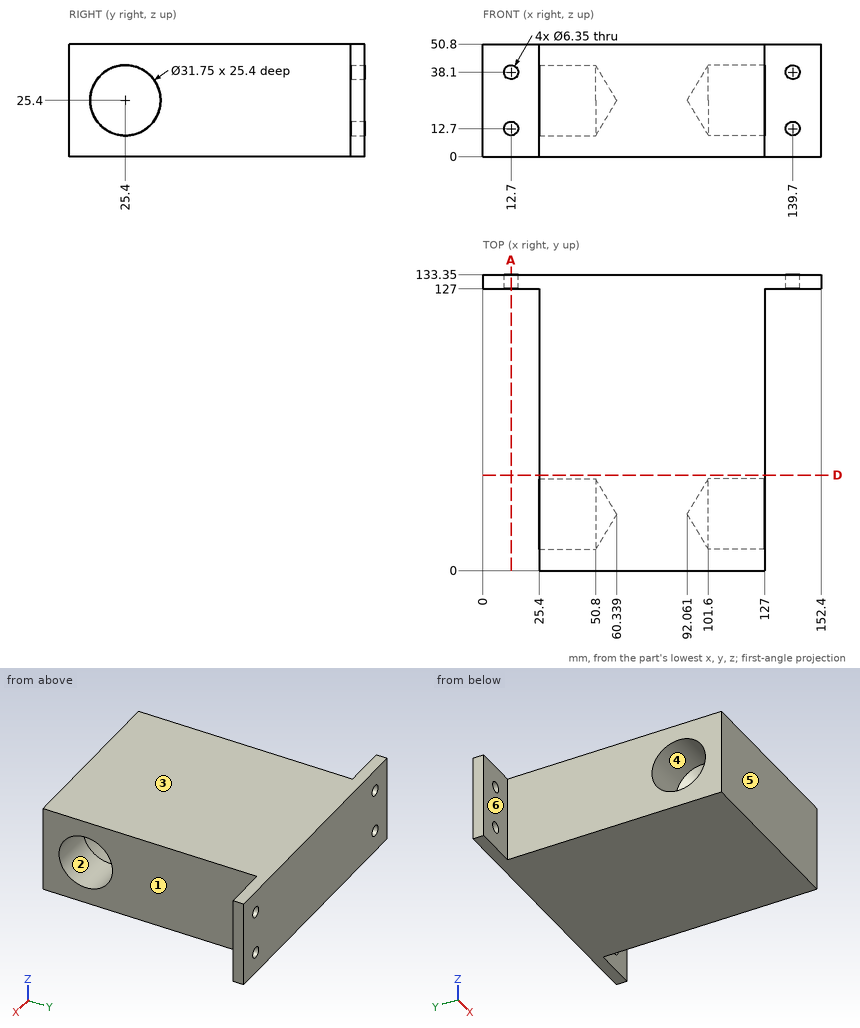
Design review of the part shown in the three views and the two pictorial views. Dimensions are in mm from the part's minimum x, y and z. A direction names the side the tool comes from. Round coordinates to 2 decimals unless told otherwise and drop trailing zeros. Order: outer loops, then holes, each group sorted by start corner. A loop starts at its lowest first (then second) coordinate and runs counter-clockwise, first axis right, second up.
(1) Take a section at A-A, the plane x = 12.7. Count the separate pieces of the cut face and the enclosed holes in it, plus the area to 3 significant figures.
Working result:
separate pieces: 3
enclosed holes: 0
area: 242 mm2
(2) Mouldability with a two-part tool opening along Z and no side actions: class the marked faces 1, 2 and 3 as released by +Z, released by -Z, zero draft, split by the parting line, or undercut.
Working result:
face 1: zero draft
face 2: undercut
face 3: released by +Z
(3) For P1, Ø6, axis at y = 105, z = 13, coming from the +X side; P2, Ø5.5, axis at x = 12.7, z = 12.7, coming from the -Y side; P3, Ø7.5, axis at x = 143.5, z = 21, coming from the -Y side; P4, Ø6, axis at x = 78.5, z = 16, coming from the -Y side, all flat-tipped, find the tip position at first contact; note any pin that passes through.
Working result:
P1: stops at x = 127
P2: passes through
P3: stops at y = 127
P4: stops at y = 0
(4) Tool access review of the marked faces 4, 5 and 6: name each direction out of +Z, -Z, +X, -X, +Y, -Y from which nothing blocks a thin tool from reaching the whole face with its end or side.
Working result:
face 4: -X
face 5: +Z, -Z, +X, -X, -Y
face 6: +Z, -Z, -X, -Y
(5) Wall thickness on L1, parallel to Z at x = 12.7, y = 130 (1 decimal); L2, parallel to Z at x = 40, y = 25; L3, parallel to Y at x = 37, z = 25: over which ranges is each line inside the solid? List them lowest first.
Working result:
L1: z = 0 to 9.5, 15.9 to 34.9, 41.3 to 50.8
L2: z = 0 to 9.53, 41.27 to 50.8
L3: y = 0 to 9.53, 41.27 to 133.35
(6) Take a section at D-D, the plane y = 43. State the section outline as (x, z) points, plus the area to 3 significant figures.
Working result:
outline: (25.4, 0) - (127, 0) - (127, 50.8) - (25.4, 50.8) - close
area: 5,160 mm2
